Work out the finished part from the listing and answer in its coordinate system (mm). Face numbers are marked on the shaded views. Round coordinates to 2 decimals unless told otherwise and drop trailing zeros. Order: outer loops, then holes, each group sorted by start corner. A loop starts at its lowest first (then second) coordinate and runs counter-clockwise, first axis right, second up. Notation, with made-up numbers: M -14.5,-7 L 29.5,-7 A24 cw 29.5,20 Z; hole C 17.5,-12 d3. An arc over 180 degrees is marked long. Return JSON: item names as keys, results as strings.
from build123d import *

# Parameters (mm, degrees)
BOSS_EXTRUDE1_DEPTH = 15.748
SKETCH2_R           = 1.905
CUT_EXTRUDE1_DEPTH  = 7.62


with BuildPart() as part:
    # Sketch1 → Boss-Extrude1 (new body)
    with BuildSketch(Plane.XY):
        with BuildLine():
            Line((-4.650037455, 0), (4.650037455, 0))
            ThreePointArc((4.650037455, 0), (4.877341219, 0.140646574), (4.852916671, 0.406826777))
            Line((4.852916671, 0.406826777), (1.905063618, 4.320133887))
            ThreePointArc((1.905063618, 4.320133887), (1.457434672, 4.692518816), (0.89066754, 4.826))
            Line((0.89066754, 4.826), (-0.89066754, 4.826))
            ThreePointArc((-0.89066754, 4.826), (-1.457434672, 4.692518816), (-1.905063618, 4.320133887))
            Line((-1.905063618, 4.320133887), (-4.852916671, 0.406826777))
            ThreePointArc((-4.852916671, 0.406826777), (-4.877341219, 0.140646574), (-4.650037455, 0))
        make_face()
    extrude(amount=-BOSS_EXTRUDE1_DEPTH)

    # Sketch2 → Cut-Extrude1 (cut)
    with BuildSketch(Plane.XZ):
        with Locations((0, -6.477)):
            Circle(SKETCH2_R)
    extrude(amount=-CUT_EXTRUDE1_DEPTH, mode=Mode.SUBTRACT)


solid = part.part
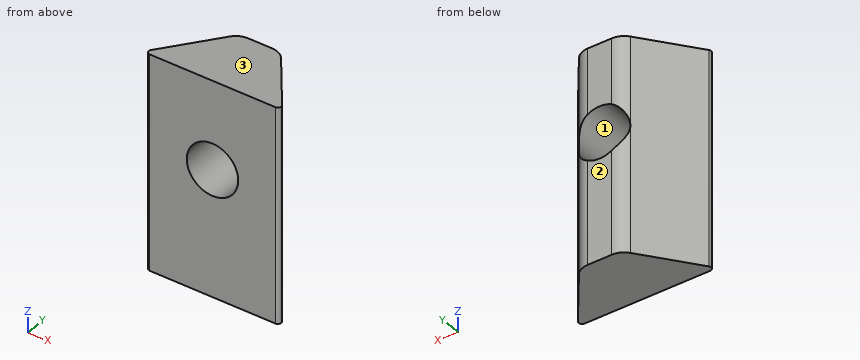
Item 1: The mould has two halves that part along Z. Classify the marked faces 1, 2 and 3: pulls with the +Z half, pulls with the -Z half, needs draft (parallel to the pull), parting line crosses it, or undercut.
Output:
{"face 1": "undercut", "face 2": "needs draft", "face 3": "pulls with the +Z half"}
Item 2: Find section B-B (z = -7). Determine the outline of the cut face in (x, y).
Output:
{"outline": "M -4.85,0.41 A0.25 ccw -4.65,0 L -1.83,0 L -1.83,4.41 A1.27 ccw -1.91,4.32 Z; M 1.83,0 L 4.65,0 A0.25 ccw 4.85,0.41 L 1.91,4.32 A1.27 ccw 1.83,4.41 Z"}
Item 3: Consider line 1 along Z through (x, y) = (0, 3.1); line 2 along Y through (x, z) = (-1, -11); line 3 along Z through (x, y) = (-1.75, 2.4). Determine where each line is inside the solid, lowest interval first. Write a range as [from, to].
Output:
{"line 1": "z = [-15.75, -8.38], [-4.57, 0]", "line 2": "y = [0, 4.82]", "line 3": "z = [-15.75, -7.23], [-5.72, 0]"}
Item 4: Each of these flat-tipped pins is pushed along its axis until it touches: pin 1 (3 mm diameter, centred on x = -3, z = -5, fed in from +Y); pin 2 (1 mm diameter, centred on y = 4, z = -8, fed in from +X). Where does it stop, or does it pass through?
Output:
{"pin 1": "stops at y = 4.67", "pin 2": "stops at x = 2.52"}
Item 5: Find section A-A (x = 0). Determine the outline of the cut face in (y, z), plus the area to 3 significant figures.
Output:
{"outline": "M 0,-15.75 L 4.83,-15.75 L 4.83,-8.38 L 0,-8.38 Z; M 0,-4.57 L 4.83,-4.57 L 4.83,0 L 0,0 Z", "area": "57.6 mm^2"}
Item 6: Find section D-D (y = 3.4). Determine the outline of the cut face in (x, z) (3 decimals).
Output:
{"outline": "M -2.598,-15.748 L 2.598,-15.748 L 2.598,0 L -2.598,0 Z; hole C 0,-6.477 d3.81"}
Item 7: Find section C-C (z = -4.25). Determine the outline of the cut face in (x, y).
Output:
{"outline": "M -4.85,0.41 A0.25 ccw -4.65,0 L 4.65,0 A0.25 ccw 4.85,0.41 L 1.91,4.32 A1.27 ccw 0.89,4.83 L -0.89,4.83 A1.27 ccw -1.91,4.32 Z"}
